Could you check a few things on this drawing? It's one solid part, dimensions in mm from its lowest x, y, z. Round coordinates to 2 decimals unless told otherwise and drop trailing zeros. Order: outer loops, then holes, each group sorted by start corner. A loop starts at its lowest first (then second) coordinate and runs counter-clockwise, first axis right, second up. Notation, with made-up numbers: (62.25, -2) - (81.25, -2) arc R14 cw to (81.25, 8) - close; hole circle Ø4 at (54, 82). An arc over 180 degrees is marked (long way). Use one line per item in the form item = value.
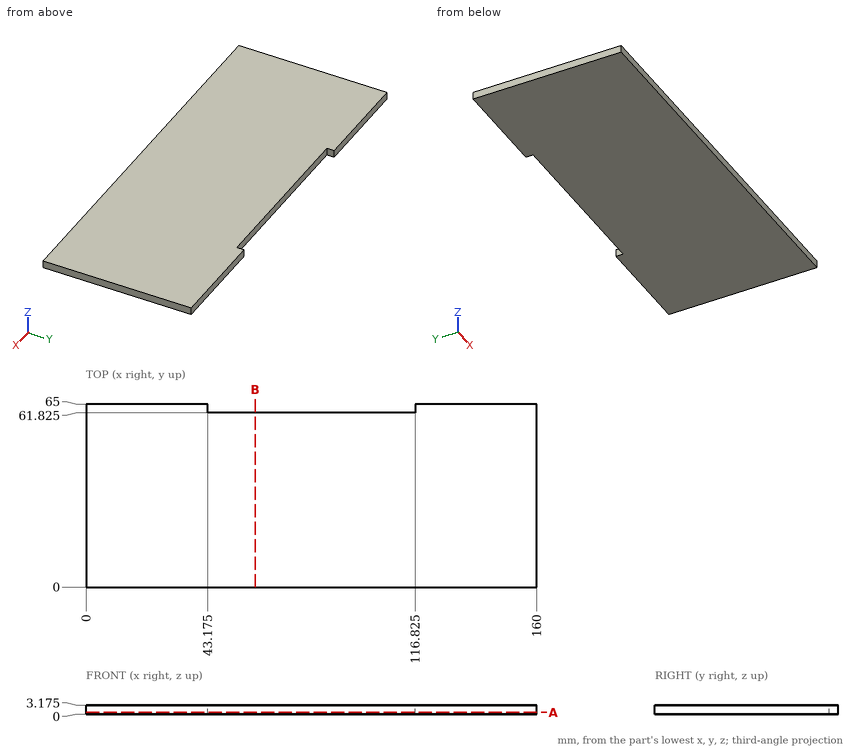
Item 1: Will these pins go through, and if not, where does the flat tip stop? P1, Ø2, axis at x = 34.5, y = 24.5, coming from the -Z side; P2, Ø1, axis at x = 73.5, z = 1.5, coming from the +Y side (3 decimals).
Found:
P1 = 0
P2 = 61.825
Item 2: Imagine slicing it at A-A on z = 0.65. Please give me the cut outline in (x, y) (3 decimals).
Found:
outline = (0, 0) - (160, 0) - (160, 65) - (116.825, 65) - (116.825, 61.825) - (43.175, 61.825) - (43.175, 65) - (0, 65) - close
Item 3: Imagine slicing it at B-B on x = 60. Please give me the cut outline in (y, z) (3 decimals), plus the area to 3 significant figures.
Found:
outline = (0, 0) - (61.825, 0) - (61.825, 3.175) - (0, 3.175) - close
area = 196 mm2
Item 4: I need wall thicknesses on L1, parallel to Y at x = 59.5, z = 1.05 (3 decimals). Which ranges of the line are inside material? Lowest first, please.
Found:
L1 = 0 to 61.825
